from build123d import *

# Parameters (mm, degrees)
SKETCH2_W               = 170
SKETCH2_H               = 170
BOSS_EXTRUDE1_DEPTH     = 10
SKETCH3_W               = 5
SKETCH3_H               = 140
SKETCH3_W_2             = 140
SKETCH3_H_2             = 4.998101886
SKETCH3_H_3             = 5
CUT_EXTRUDE1_DEPTH      = 10
CUT_EXTRUDE2_DEPTH      = 121.623380818
CUT_EXTRUDE2_DEPTH_BACK = 121.623380818
SKETCH4_R               = 1.5


with BuildPart() as part:
    # Sketch2 → Boss-Extrude1 (new body)
    with BuildSketch(Plane(origin=(0, 0, 0), x_dir=(1, 0, 0), z_dir=(0, 1, 0))):
        Rectangle(SKETCH2_W, SKETCH2_H)
    extrude(amount=BOSS_EXTRUDE1_DEPTH)

    # Sketch3 → Cut-Extrude1 (cut)
    with BuildSketch(Plane(origin=(0, 10, 0), x_dir=(1, 0, 0), z_dir=(0, 1, 0))):
        with Locations((-77.5, 0)):
            Rectangle(SKETCH3_W, SKETCH3_H)
        with Locations((0, -77.500949057)):
            Rectangle(SKETCH3_W_2, SKETCH3_H_2)
        with Locations((77.5, 0)):
            Rectangle(SKETCH3_W, SKETCH3_H)
        with Locations((0, 77.5)):
            Rectangle(SKETCH3_W_2, SKETCH3_H_3)
    extrude(amount=-CUT_EXTRUDE1_DEPTH, mode=Mode.SUBTRACT)

    # Sketch4 → Cut-Extrude2 (cut, two sides: drawn at the far end of the back side and taken through both)
    with BuildSketch(Plane(origin=(0, 0, 0), x_dir=(-1, 0, 0), z_dir=(0, -1, 0)).offset(-CUT_EXTRUDE2_DEPTH_BACK)):
        with Locations(Location((-70.33, -9, 0), (0, 0, 270))):
            Circle(SKETCH4_R)
        with Locations(Location((-70.33, 9, 0), (0, 0, 270))):
            Circle(SKETCH4_R)
        with Locations(Location((70.33, 9, 0), (0, 0, 270))):
            Circle(SKETCH4_R)
        with Locations(Location((70.33, -9, 0), (0, 0, 270))):
            Circle(SKETCH4_R)
        with Locations(Location((46.4, 9, 0), (0, 0, 270))):
            Circle(SKETCH4_R)
        with Locations(Location((46.4, -9, 0), (0, 0, 270))):
            Circle(SKETCH4_R)
        with Locations(Location((-46.4, -9, 0), (0, 0, 270))):
            Circle(SKETCH4_R)
        with Locations(Location((-46.4, 9, 0), (0, 0, 270))):
            Circle(SKETCH4_R)
    extrude(amount=CUT_EXTRUDE2_DEPTH + CUT_EXTRUDE2_DEPTH_BACK, mode=Mode.SUBTRACT)


solid = part.part
Design review of the part built by this model. Coordinates are the model's own, in mm. A direction names the side the tool comes from. Round coordinates to 2 decimals unless told otherwise and drop trailing zeros. Write each loop counter-clockwise with the first axis right and the second up, starting at its lowest first coordinate (ties: lowest second). Pieces come first, ordered by that corner, then holes. Notation, with made-up numbers: (81, 87.25) -> (102, 87.25) arc R23 ccw to (102, 105.25) -> close; hole circle Ø6 at (20.25, -37.75). An arc over 180 degrees is marked (long way). One line per item, written item: value. Start each with the question number.
Q1. Add section A-A (x = -33.5). Give the boundary of the cut face in (y, z).
Q2. To check wall thickness, follow probe 1 along Z at (x, y) = (30, 3.5); probe 2 along Z at (x, y) = (-70.33, 5.5). State the ranges of each line that lie inside material, in increasing order.
Q3. Add section C-C (y = 5.5). State how many separate pieces and enclosed holes the cut face has, then the cut area to 3 significant figures.
Q4. Tool access review of faces 5 (the face through (-70, 5, 78)), 6 (the face through (-1, 5, -85)): name each direction out of +Z, -Z, +X, -X, +Y, -Y from which nothing blocks a thin tool from reaching the whole face with its end or side.
Q5. Add section B-B (z = -60.5). Give the boundary of the cut face in (x, y), then the cut area to 3 significant figures.
Q6. The part is to be moulded in two halves that separate along X. For faces 1 (the face through (70, 5, 78)), 2 (the face through (85, 5, 1)), 3 (the face through (-1, 0, -1)), 4 (the face through (-78, 5, 70)), say which applies: pulls with the +X half, pulls with the -X half, needs draft (parallel to the pull), parting line crosses it, or undercut.
Response:
1. outline: (0, -85) -> (10, -85) -> (10, -80) -> (0, -80) -> close; (0, -75) -> (10, -75) -> (10, 75) -> (0, 75) -> close; (0, 80) -> (10, 80) -> (10, 85) -> (0, 85) -> close
2. probe 1: z = -85 to -80, -75 to 75, 80 to 85
2. probe 2: z = -85 to -10.5, -7.5 to 7.5, 10.5 to 85
3. separate pieces: 1
3. enclosed holes: 12
3. area: 26,000 mm^2
4. face 5: +Y, -Y
4. face 6: -Z, +X, -X, +Y, -Y
5. outline: (-85, 0) -> (-80, 0) -> (-80, 10) -> (-85, 10) -> close; (-75, 0) -> (75, 0) -> (75, 10) -> (-75, 10) -> close; (80, 0) -> (85, 0) -> (85, 10) -> (80, 10) -> close
5. area: 1,600 mm^2
6. face 1: undercut
6. face 2: pulls with the +X half
6. face 3: needs draft
6. face 4: undercut
